Geometry: final body of the model. Coordinates: model frame, mm. Give positions to 0.01 mm unless a question says otherwise; leave off trailing zeros. Write each loop counter-clockwise with the first axis right and the second up, starting at its lowest first coordinate (ties: lowest second). Pieces come first, ordered by that corner, then holes. Notation, with made-up numbers: (-29, -38.75) - (-5, -38.75) arc R23 cw to (-5, -25.75) - close; hole circle Ø5 at (-25, -20.5). An arc over 180 degrees is marked (long way). Return JSON: item names as keys, results as strings.
from build123d import *

# Parameters (mm, degrees)
SKETCH_1_R      = 3
SKETCH_1_W      = 30
SKETCH_1_H      = 5
SKETCH_1_W_2    = 5
SKETCH_1_H_2    = 15
SKETCH_1_W_3    = 10
SKETCH_1_H_3    = 3.5
SKETCH_1_W_4    = 41
SKETCH_1_H_4    = 7.3
EXTRUDE_1_DEPTH = 5


with BuildPart() as part:
    # 草图1 → 凸台-拉伸1 (new body)
    with BuildSketch(Plane.XY):
        with BuildLine():
            Line((0, 0), (-80, 0))
            Line((-80, 0), (-80, 13))
            Line((-80, 13), (-77.5, 13))
            Line((-77.5, 13), (-77.5, 53))
            Line((-77.5, 53), (-54, 53))
            ThreePointArc((-54, 53), (-51.171572875, 51.828427125), (-50, 49))
            Line((-50, 49), (-50, 48))
            Line((-50, 48), (-30, 48))
            Line((-30, 48), (-30, 49))
            ThreePointArc((-30, 49), (-28.828427125, 51.828427125), (-26, 53))
            Line((-26, 53), (-2.5, 53))
            Line((-2.5, 53), (-2.5, 13))
            Line((-2.5, 13), (0, 13))
            Line((0, 13), (0, 0))
        make_face()
        with Locations((-68.55, 47)):
            Circle(SKETCH_1_R, mode=Mode.SUBTRACT)
        with Locations((-11.45, 47)):
            Circle(SKETCH_1_R, mode=Mode.SUBTRACT)
        with Locations((-40, 43)):
            Rectangle(SKETCH_1_W, SKETCH_1_H, mode=Mode.SUBTRACT)
        with Locations((-67.5, 23)):
            Rectangle(SKETCH_1_W_2, SKETCH_1_H_2, mode=Mode.SUBTRACT)
        with Locations((-12.5, 23)):
            Rectangle(SKETCH_1_W_2, SKETCH_1_H_2, mode=Mode.SUBTRACT)
        Polygon((-55, 16), (-50, 16), (-30, 16), (-25, 16), (-25, 21), (-55, 21), align=None, mode=Mode.SUBTRACT)
        with Locations((-57.5, 11.5)):
            Rectangle(SKETCH_1_W_2, SKETCH_1_H, mode=Mode.SUBTRACT)
        with Locations((-22.5, 11.5)):
            Rectangle(SKETCH_1_W_2, SKETCH_1_H, mode=Mode.SUBTRACT)
        with Locations((-40, 10.75)):
            Rectangle(SKETCH_1_W_3, SKETCH_1_H_3, mode=Mode.SUBTRACT)
        with Locations((-42.5, 34.15)):
            Rectangle(SKETCH_1_W_4, SKETCH_1_H_4, mode=Mode.SUBTRACT)
    extrude(amount=EXTRUDE_1_DEPTH)


solid = part.part
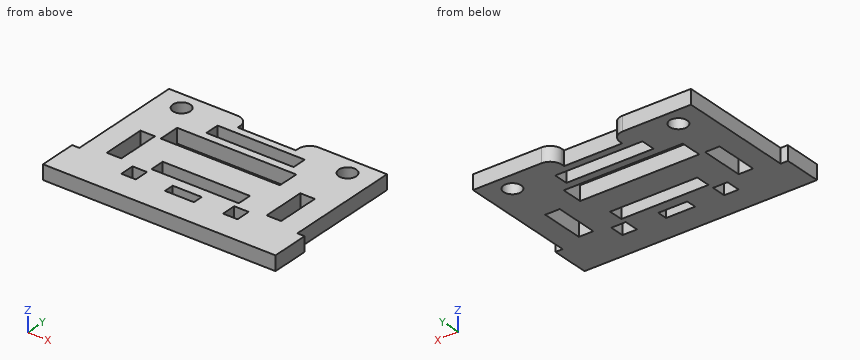
Q1. Material intervals for probe 1 along X at (y, z) = (18, 3.25); probe 2 along Y at (x, z) = (-48, 0.3); probe 3 along Y at (x, z) = (-11.45, 1.85), sorted ascending. Write a range as [from, to].
Answer key:
{"probe 1": "x = [-77.5, -70], [-65, -55], [-25, -15], [-10, -2.5]", "probe 2": "y = [0, 16], [21, 30.5], [37.8, 40.5], [45.5, 48]", "probe 3": "y = [0, 15.5], [30.5, 44], [50, 53]"}
Q2. Section query D-D, the plane x = -33.5. Return the cut outline in (y, z), plus the area to 4 significant figures.
Answer key:
{"outline": "(0, 0) - (16, 0) - (16, 5) - (0, 5) - close; (21, 0) - (30.5, 0) - (30.5, 5) - (21, 5) - close; (37.8, 0) - (40.5, 0) - (40.5, 5) - (37.8, 5) - close; (45.5, 0) - (48, 0) - (48, 5) - (45.5, 5) - close", "area": "153.5 mm^2"}
Q3. Section query C-C, the plane y = 10. Return the cut outline in (x, z).
Answer key:
{"outline": "(-80, 0) - (-60, 0) - (-60, 5) - (-80, 5) - close; (-55, 0) - (-45, 0) - (-45, 5) - (-55, 5) - close; (-35, 0) - (-25, 0) - (-25, 5) - (-35, 5) - close; (-20, 0) - (0, 0) - (0, 5) - (-20, 5) - close"}
Q4. Pin query (flat end, axial travel): P1, Ø1.5, axis at x = -44.5, z = 3.5, coming from the +Y side; P2, Ø0.8, axis at y = 48.5, z = 2.5, coming from the -X side; P3, Ø3, axis at x = -79.5, z = 3, coming from the +Y side; P4, Ø1, axis at y = 11, z = 3, coming from the +X side. Return the tip coordinate at first contact, or that it passes through.
Answer key:
{"P1": "stops at y = 48", "P2": "stops at x = -77.5", "P3": "stops at y = 13", "P4": "stops at x = 0"}
Q5. Section query B-B, the plane x = -68.55. Return the cut outline in (y, z), plus the area to 3 significant figures.
Answer key:
{"outline": "(0, 0) - (15.5, 0) - (15.5, 5) - (0, 5) - close; (30.5, 0) - (44, 0) - (44, 5) - (30.5, 5) - close; (50, 0) - (53, 0) - (53, 5) - (50, 5) - close", "area": "160 mm^2"}
Q6. Section query A-A, the plane y = 47. Return the cut outline in (x, z), plus the area to 3 significant figures.
Answer key:
{"outline": "(-77.5, 0) - (-71.55, 0) - (-71.55, 5) - (-77.5, 5) - close; (-65.55, 0) - (-14.45, 0) - (-14.45, 5) - (-65.55, 5) - close; (-8.45, 0) - (-2.5, 0) - (-2.5, 5) - (-8.45, 5) - close", "area": "315 mm^2"}
